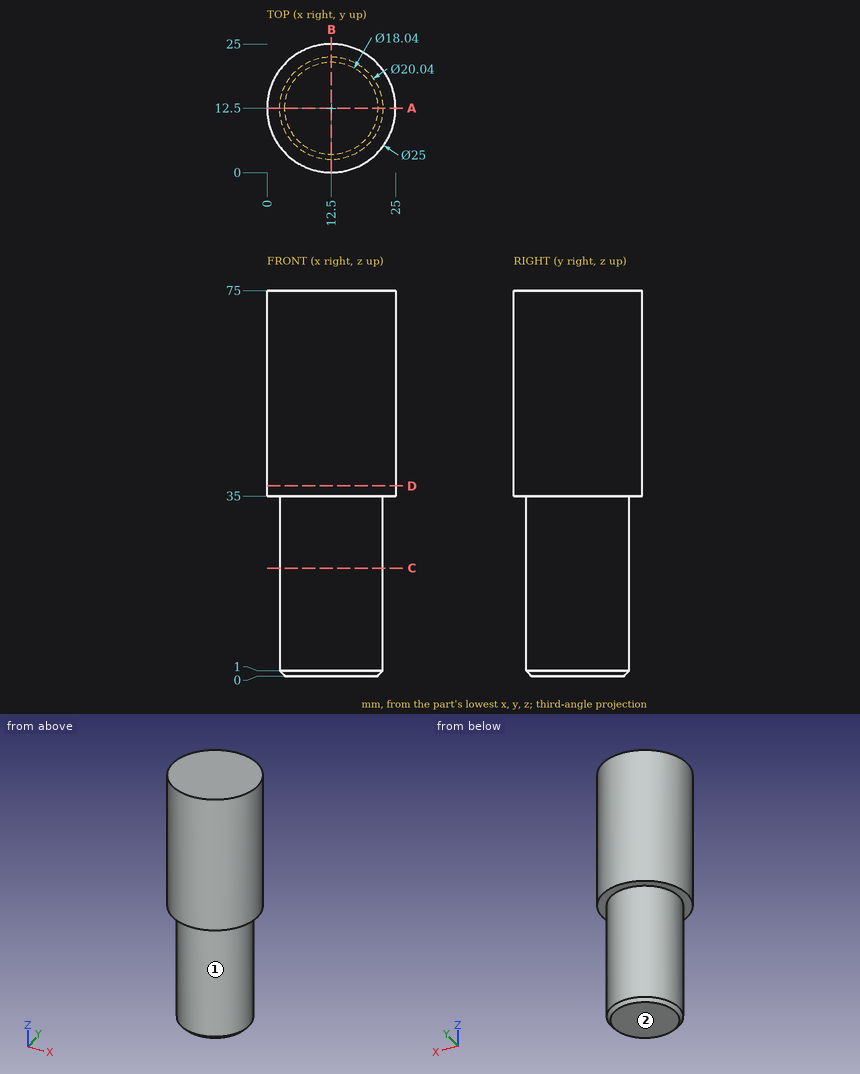
Could you check a few things on this drawing? It's one solid part, dimensions in mm from its lowest x, y, z. A direction names the side the tool comes from. Round coordinates to 2 decimals unless told otherwise and drop trailing zeros. Order: outer loops, then holes, each group sorted by start corner. A loop starts at its lowest first (then second) coordinate and runs counter-clockwise, first axis right, second up. Notation, with made-up numbers: M -14,26 L 39,26 A23 ccw 39,45 Z; hole C 14.25,-6 d8. An arc over 180 degrees is marked long. Return JSON: item names as keys, results as strings. Group by question number.
1. On a 3-axis mill with a long thin cutter (end or side, diameter ignored), from which of +Z, -Z, +X, -X, +Y, -Y can I reach the whole of each face in a straight line? I mean the marked faces 1 and 2. Say none if no direction works.
2. Please list where these lines run through material, in increasing order: probe 1 along Z at (x, y) = (23.5, 8.5); probe 2 along Y at (x, z) = (13, 35.5); probe 3 along Y at (x, z) = (13, 22).
3. If we section it at D-D on z = 37: List the corners of the cut face in (x, y) for me.
4. If we section it at C-C on z = 21: List the corners of the cut face in (x, y) for me, then the cut area to 3 significant figures.
5. If we section it at A-A on y = 12.5: List the corners of the cut face in (x, z) for me, then the cut area to 3 significant figures.
6. I'm going to push flat-ended pins straight in: pin 1 Ø8 at (x, z) = (4.5, 51.5) entering from +Y; pin 2 Ø6 at (y, z) = (11, 39) entering from -X; pin 3 Ø8 at (x, z) = (3, 51.5) entering from -Y (3 decimals); pin 4 Ø1.5 at (x, y) = (3, 4) entering from -Z. Where does each tip first touch, or does it pass through?
Reply:
{
 "1": {"face 1": "-Z", "face 2": "-Z, +X, -X, +Y, -Y"},
 "2": {"probe 1": "35 to 75", "probe 2": "0.01 to 24.99", "probe 3": "2.49 to 22.51"},
 "3": {"outline": "C 12.5,12.5 d25"},
 "4": {"outline": "C 12.5,12.5 d20.04", "area": "315 mm^2"},
 "5": {"outline": "M 0,35 L 2.48,35 L 2.48,1 L 3.48,0 L 21.52,0 L 22.52,1 L 22.52,35 L 25,35 L 25,75 L 0,75 Z", "area": "1,700 mm^2"},
 "6": {"pin 1": "y = 24.34", "pin 2": "x = 0", "pin 3": "y = 1.275", "pin 4": "z = 35"}
}
